The listing builds one solid part. Answer for the finished solid, in the listing's coordinates (mm). A direction names the side the tool comes from. Coordinates: 2 decimals unless noted, no trailing zeros. Write each loop counter-clockwise with the first axis right and the second up, starting at its lowest first coordinate (ties: lowest second). Pieces come first, ordered by that corner, then holes. Notation, with made-up numbers: M 64.25,28 L 85.25,28 A21 ccw 85.25,49 Z; hole C 29.25,-0.5 d10. An arc over 180 degrees is marked long. Put each result on its own line as item: value. Start each with the question number.
```python
from build123d import *

# Parameters (mm, degrees)
BRIDA_BASE1_DEPTH                = 2
BRIDA_DE_ARISTA1_STRIP_W         = 9.4732
BRIDA_DE_ARISTA1_STRIP_H         = 2
BRIDA_DE_ARISTA1_STRIP_CUT_DEPTH = 87.5
BRIDA_DE_ARISTA1_DEPTH           = 87.5
BRIDA_DE_ARISTA2_STRIP_W         = 9.4732
BRIDA_DE_ARISTA2_STRIP_H         = 2
BRIDA_DE_ARISTA2_STRIP_CUT_DEPTH = 431.2634
BRIDA_DE_ARISTA2_DEPTH           = 431.2634
BRIDA_DE_ARISTA3_STRIP_W         = 9.4732
BRIDA_DE_ARISTA3_STRIP_H         = 2
BRIDA_DE_ARISTA3_STRIP_CUT_DEPTH = 135.2634
BRIDA_DE_ARISTA3_DEPTH           = 135.2634


# Sheet-metal steps are written as plain solids
with BuildPart() as part:
    # Croquis1 → Brida base1 (new body)
    with BuildSketch(Plane(origin=(0, 0, 0), x_dir=(1, 0, 0), z_dir=(0, 1, 0))):
        Polygon((-67, -69), (217, -69), (217, 69), (-217, 69), (-217, -18.5), (-67, -18.5), align=None)
    extrude(amount=-BRIDA_BASE1_DEPTH)

    # Brida de arista1 strip (across the edge) → Brida de arista1 strip cut (cut)
    with BuildSketch(Plane(origin=(-217, 0, -69), x_dir=(1, 0, 0), z_dir=(0, 0, 1))):
        with Locations((-2, -1)):
            Rectangle(BRIDA_DE_ARISTA1_STRIP_W, BRIDA_DE_ARISTA1_STRIP_H)
    extrude(amount=BRIDA_DE_ARISTA1_STRIP_CUT_DEPTH, mode=Mode.SUBTRACT)

    # Brida de arista1 section (across the edge) → Brida de arista1 (add)
    with BuildSketch(Plane(origin=(-217, 0, -69), x_dir=(1, 0, 0), z_dir=(0, 0, 1))):
        with BuildLine():
            Line((0, 0.7366), (0, 46))
            Line((0, 46), (2, 46))
            Line((2, 46), (2, 0.7366))
            ThreePointArc((2, 0.7366), (2.215745145, 0.215745145), (2.7366, 0))
            Line((2.7366, 0), (2.7366, -2))
            ThreePointArc((2.7366, -2), (0.801531583, -1.198468417), (0, 0.7366))
        make_face()
    extrude(amount=BRIDA_DE_ARISTA1_DEPTH)

    # Brida de arista2 strip (across the edge) → Brida de arista2 strip cut (cut)
    with BuildSketch(Plane(origin=(217, 0, -69), x_dir=(0, 0, 1), z_dir=(-1, 0, 0))):
        with Locations((-2, -1)):
            Rectangle(BRIDA_DE_ARISTA2_STRIP_W, BRIDA_DE_ARISTA2_STRIP_H)
    extrude(amount=BRIDA_DE_ARISTA2_STRIP_CUT_DEPTH, mode=Mode.SUBTRACT)

    # Brida de arista2 section (across the edge) → Brida de arista2 (add)
    with BuildSketch(Plane(origin=(217, 0, -69), x_dir=(0, 0, 1), z_dir=(-1, 0, 0))):
        with BuildLine():
            Line((0, 0.7366), (0, 46))
            Line((0, 46), (2, 46))
            Line((2, 46), (2, 0.7366))
            ThreePointArc((2, 0.7366), (2.215745145, 0.215745145), (2.7366, 0))
            Line((2.7366, 0), (2.7366, -2))
            ThreePointArc((2.7366, -2), (0.801531583, -1.198468417), (0, 0.7366))
        make_face()
    extrude(amount=BRIDA_DE_ARISTA2_DEPTH)

    # Brida de arista3 strip (across the edge) → Brida de arista3 strip cut (cut)
    with BuildSketch(Plane(origin=(217, 0, 69), x_dir=(-1, 0, 0), z_dir=(0, 0, -1))):
        with Locations((-2, -1)):
            Rectangle(BRIDA_DE_ARISTA3_STRIP_W, BRIDA_DE_ARISTA3_STRIP_H)
    extrude(amount=BRIDA_DE_ARISTA3_STRIP_CUT_DEPTH, mode=Mode.SUBTRACT)

    # Brida de arista3 section (across the edge) → Brida de arista3 (add)
    with BuildSketch(Plane(origin=(217, 0, 69), x_dir=(-1, 0, 0), z_dir=(0, 0, -1))):
        with BuildLine():
            Line((0, 0.7366), (0, 46))
            Line((0, 46), (2, 46))
            Line((2, 46), (2, 0.7366))
            ThreePointArc((2, 0.7366), (2.215745145, 0.215745145), (2.7366, 0))
            Line((2.7366, 0), (2.7366, -2))
            ThreePointArc((2.7366, -2), (0.801531583, -1.198468417), (0, 0.7366))
        make_face()
    extrude(amount=BRIDA_DE_ARISTA3_DEPTH)


solid = part.part
```
1) A cutting plane is placed at B-B on y = 41.5. Write down the section's boundary in (x, z), then the cut area to 3 significant figures.
2) Given pin 1 Ø22.5 at (x, y) = (89, 12.5) entering from +Z; pin 2 Ø4 at (x, z) = (-169, -37) entering from +Y; pin 3 Ø1 at (y, z) = (-1, 46) entering from -X, each flat-ended and moving along its own axis, determine where each tip first touches the part or whether it passes through.
3) A cutting plane is placed at C-C on x = 166. Write down the section's boundary in (y, z).
4) Straight lines are drawn through the part: probe 1 along X at (y, z) = (17.5, -13.5); probe 2 along Y at (x, z) = (75.5, -38); probe 3 along Z at (x, y) = (45, 24.5). For each, find the intervals that lie inside material, in ascending order.
5) A cutting plane is placed at D-D on z = -17.5. Write down the section's boundary in (x, y).
6) Determine the mould class of faces 1 (the face through (74, -1, 69)), 2 (the face through (217, 23, 2)), 3 (the face through (-215, 24, -26)) for opening direction X: +X half, -X half, draft (parallel to the pull), parting line (faces both ways), or undercut.
7) A cutting plane is placed at A-A on z = 51.5. Write down the section's boundary in (x, y).
8) For faces 4 (the face through (-142, -1, 18.5)), 5 (the face through (4, 23, -69)), 6 (the face through (215, 24, 2)), determine the directions among +Z, -Z, +X, -X, +Y, -Y from which every point of the face is accessible in a straight line to the end or side of a thin tool.
Answers follow:
1. outline: M -217,-69 L -215,-69 L -215,18.5 L -217,18.5 Z; M -214.26,-69 L 217,-69 L 217,-67 L -214.26,-67 Z; M 215,-66.26 L 217,-66.26 L 217,69 L 215,69 Z
1. area: 1,310 mm²
2. pin 1: stops at z = -67
2. pin 2: stops at y = 0
2. pin 3: stops at x = -67
3. outline: M -2,-66.26 A2.74 ccw 0.74,-69 L 46,-69 L 46,-67 L 0.74,-67 A0.74 cw 0,-66.26 L 0,69 L -2,69 Z
4. probe 1: x = -217 to -215, 215 to 217
4. probe 2: y = -2 to 0
4. probe 3: z = -69 to -67
5. outline: M -217,0.74 A2.74 ccw -214.26,-2 L 214.26,-2 A2.74 ccw 217,0.74 L 217,46 L 215,46 L 215,0.74 A0.74 cw 214.26,0 L -214.26,0 A0.74 cw -215,0.74 L -215,46 L -217,46 Z
6. face 1: draft
6. face 2: +X half
6. face 3: undercut
7. outline: M -67,-2 L 214.26,-2 A2.74 ccw 217,0.74 L 217,46 L 215,46 L 215,0.74 A0.74 cw 214.26,0 L -67,0 Z
8. face 4: +Z, -X, +Y, -Y
8. face 5: -Z, +X, -X, +Y, -Y
8. face 6: +Z, +Y
